from build123d import *

# Parameters (mm, degrees)
F1_DEPTH = 13
F2_R     = 1.99999


# Not quite as in the source:
# - a fillet or chamfer is up to 0.001 mm smaller than in the source, because OpenCascade refuses the exact size


with BuildPart() as f1:
    # F0 (on Top) → F1 (new body)
    with BuildSketch(Plane.XY):
        with BuildLine():
            Line((0, 10), (0, 24.5))
            Line((0, 24.5), (-2, 24.5))
            Line((-2, 24.5), (-2, 4.5))
            ThreePointArc((-2, 4.5), (2.5, 0), (7, 4.5))
            ThreePointArc((7, 4.5), (6.2015841123, 9.9720743607), (3.8729089523, 14.9878831427))
            ThreePointArc((3.8729089523, 14.9878831427), (3.7530227087, 17.0940905495), (5.2871913605, 18.5421267712))
            ThreePointArc((5.2871913605, 18.5421267712), (5.3073257689, 18.5487259027), (5.3275153833, 18.5551541535))
            ThreePointArc((5.3275153833, 18.5551541535), (5.9849559235, 19.6728057544), (4.9863180052, 20.4999063971))
            ThreePointArc((4.9863180052, 20.4999063971), (4.6777817893, 20.4017930021), (4.3769319754, 20.2821676525))
            ThreePointArc((4.3769319754, 20.2821676525), (1.9143946428, 17.6625142897), (2.0963385188, 14.0717524929))
            ThreePointArc((2.0963385188, 14.0717524929), (2.172582587, 13.95665433), (2.2479018586, 13.8409488747))
            ThreePointArc((2.2479018586, 13.8409488747), (4.2976593275, 9.3689672945), (5, 4.5))
            ThreePointArc((5, 4.5), (2.5, 2), (0, 4.5))
            Line((0, 4.5), (0, 10))
        make_face()
    extrude(amount=F1_DEPTH)

    # F2 (radius 2 in the source; OpenCascade refuses exactly that, so slightly less here)
    f2_edges = [f1.edges().sort_by_distance(p)[0] for p in [
        (0, 24.5, 6.5),
    ]]
    fillet(f2_edges, radius=F2_R)


solid = f1.part
Design review of the part built by this model. Coordinates are the model's own, in mm. A direction names the side the tool comes from. Round coordinates to 2 decimals unless told otherwise and drop trailing zeros. Loops run counter-clockwise (first coordinate to the right, second up) from the corner with the lowest first, then second, coordinate; pieces in that order, holes last. Notation, with made-up numbers: (50.5, 45) - (88.5, 45) arc R4 ccw to (88.5, 49) - close; hole circle Ø2 at (50, 74.25). An arc over 180 degrees is marked (long way). One line per item, written item: value. Start each with the question number.
1) Insertion check: pin 1 Ø6.5 at (y, z) = (17, 9.5) entering from +X; pin 2 Ø3 at (y, z) = (11.5, 9) entering from +X; pin 3 Ø1 at (x, z) = (3, 8.5) entering from +Y (3 decimals). Each pin has a flat end and moves straight along its axis. Give the tip position at first contact, or say it passes through.
2) Consider section C-C on x = 3. Give the boundary of the cut face in (y, z), then the cut area to 3 significant figures.
3) For faces 4 (the cylindrical face through (-0.6, 23.93, 6.59)), 5 (the flat face through (0, 13, 6)), 6 (the cylindrical face through (6.224, 9.898, 6.409)), list the 3-axis set-ups (+Z, -Z, +X, -X, +Y, -Y) from which the entire face can be reached by the end or side of a thin tool; tool diameter is ignored.
4) Consider section D-D on y = 20.75. Give the boundary of the cut face in (x, z).
5) To check wall thickness, follow L1, parallel to X at y = 16, z = 11.5; L2, parallel to Y at x = 2, z = 2.5; L3, parallel to X at y = 10.5, z = 8.5. State the ranges of each line that lie inside material, in increasing order. Write a range as from..to.
6) Consider section B-B on y = 6.25. Give the boundary of the cut face in (x, z), then the cut area to 3 significant figures.
7) Draft analysis for pull direction Y (two halves, no side actions). For faces 1 (the flat face through (-2, 15, 6)), 2 (the cylindrical face through (2.6, 2, 6.4)), 3 (the cylindrical face through (2.4, 0, 6.4)), state which applies: +Y half, -Y half, draft (parallel to the pull), parting line (faces both ways), or undercut.
Reported:
1. pin 1: stops at x = 6
1. pin 2: stops at x = 6.19
1. pin 3: stops at y = 19.775
2. outline: (0.03, 0) - (2.05, 0) - (2.05, 13) - (0.03, 13) - close; (12.56, 0) - (19.35, 0) - (19.35, 13) - (12.56, 13) - close
2. area: 115 mm^2
3. face 4: +Z, -Z, +X, +Y
3. face 5: +Z, -Z, +Y
3. face 6: +Z, -Z, +X
4. outline: (-2, 0) - (0, 0) - (0, 13) - (-2, 13) - close
5. L1: x = -2..0, 1.63..3.58
5. L2: y = 0.03..2.05, 14.28..17.88
5. L3: x = -2..0, 3.92..6.04
6. outline: (-2, 0) - (0, 0) - (0, 13) - (-2, 13) - close; (4.91, 0) - (6.92, 0) - (6.92, 13) - (4.91, 13) - close
6. area: 52.1 mm^2
7. face 1: draft
7. face 2: undercut
7. face 3: -Y half
